Can you work these out from the model? Positions are in its coordinate system, mm. Round coordinates to 2 decimals unless told otherwise and drop trailing zeros. Write each loop counter-clockwise with the first axis right and the second up, starting at its lowest first coordinate (ties: lowest second). Pieces come first, ordered by that corner, then holes. Notation, with made-up numbers: M -22.5,-36.5 L 21.5,-36.5 A17 ccw 21.5,-25.5 Z; hole C -23.5,62.5 d11. An arc over 180 degrees is marked long. Answer as a JSON object with one key per item and string values. Group by question number.
1) Please list where these lines run through material, in increasing order: L1, parallel to Z at x = 30.5, y = 15.5; L2, parallel to Y at x = -18, z = 19.5; L3, parallel to Y at x = 4.5, z = 17. Write a range as [from, to].
2) I'm going to push flat-ended pins straight in: pin 1 Ø2 at (x, y) = (2, 8.5) entering from +Z; pin 2 Ø4 at (x, y) = (-14.5, 36.5) entering from -Z; pin 3 Ø1 at (x, y) = (-19, 50.5) entering from +Z. Where does each tip first touch, or does it pass through?
3) Suppose I cut it at A-A, the plane y = 36.5. Write out the boundary of the cut face in (x, z) (1 decimal).
Autodesk Inventor part; units mm, degrees
ref_plane "YZ Plane" through (0, 0, 0) normal (1, 0, 0) x (0, 1, 0)
ref_plane "XZ Plane" through (0, 0, 0) normal (0, 1, 0) x (-1, 0, 0)
ref_plane "XY Plane" through (0, 0, 0) normal (0, 0, 1) x (1, 0, 0)
sketch "Sketch1" plane through (0, 0, 0) normal (0, 0, 1) x (1, 0, 0)
  line L0 (0, 0) -> (40, 0)
  arc A0 (0, -9.4427) -> (40, 0) centre (0, 80) ccw
  line L1 (40, 0) -> (30, 80)
  line L2 (30, 80) -> (0, 80)
  line L3 (0, 80) -> (0, -9.4427)
  dimension "d0" = 40
  dimension "d1" = 80
  dimension "d2" = 30
revolve "Revolution1" add sketch "Sketch1" angle 360 about axis through (0, 80, 0) along (0, -1, 0)
fillet "Fillet1" radius 20 1 edges at (-30, 80, 0)
chamfer "Chamfer1" distance 10 distance2 20 1 edges at (-40, 0, 0) measured on face at (-36.1941, -1.4854, 7.0791)
fillet "Fillet2" radius 20 1 edges at (-30.8197, -3.9651, 0)
fillet "Fillet3" radius 60 1 edges at (-37.5193, 19.8456, 0)
properties part number "body_ref"
Results:
{
 "1": {"L1": "[-18.77, 18.77]", "L2": "[-3.92, 74.09]", "L3": "[-7.7, 79.3]"},
 "2": {"pin 1": "z = 34.54", "pin 2": "z = -33.21", "pin 3": "z = 28.16"},
 "3": {"outline": "C 0,0 d70.9"}
}
